The figure shows three views and two pictorial views of one solid part (mm, origin at its lowest corner). Answer the questions. Coordinates: 2 decimals unless noted, no trailing zeros. Loops run counter-clockwise (first coordinate to the right, second up) from the corner with the lowest first, then second, coordinate; pieces in that order, holes last.
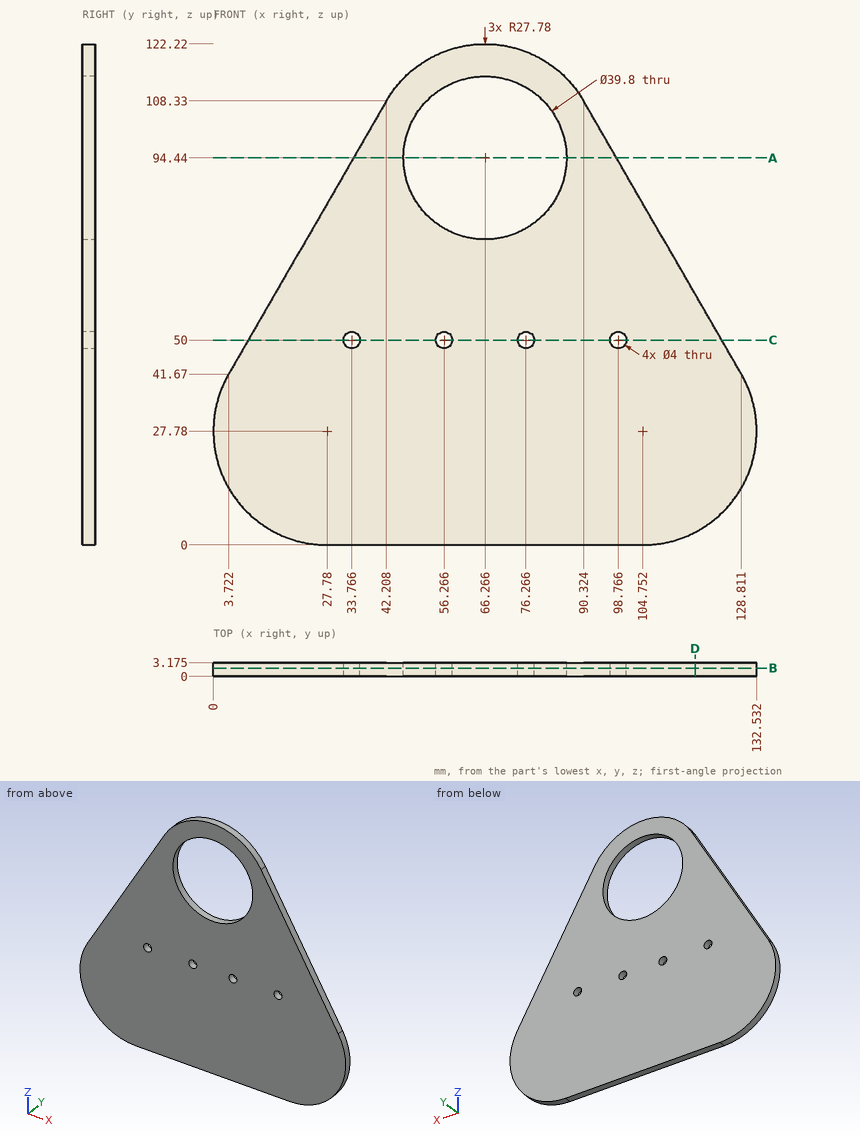
Q1. A cutting plane is placed at A-A (z = 94.44). Give the vertices of the cut face in (x, y) (1 decimal).
Findings below:
outline: (34.2, 0) - (46.4, 0) - (46.4, 3.2) - (34.2, 3.2) - close; (86.2, 0) - (98.3, 0) - (98.3, 3.2) - (86.2, 3.2) - close
Q2. A flat-ended cylindrical pin translates along its axis: pin 1 Ø1.5 at (x, y) = (74.5, 1.5) entering from +Z. Find the tip coordinate at first contact, or state that the pin passes through.
Findings below:
pin 1: stops at z = 121.19
Q3. A cutting plane is placed at C-C (z = 50). Give the vertices of the cut face in (x, y) (1 decimal), then the cut area to 3 significant figures.
Findings below:
outline: (8.5, 0) - (31.8, 0) - (31.8, 3.2) - (8.5, 3.2) - close; (35.8, 0) - (54.3, 0) - (54.3, 3.2) - (35.8, 3.2) - close; (58.3, 0) - (74.3, 0) - (74.3, 3.2) - (58.3, 3.2) - close; (78.3, 0) - (96.8, 0) - (96.8, 3.2) - (78.3, 3.2) - close; (100.8, 0) - (124, 0) - (124, 3.2) - (100.8, 3.2) - close
area: 316 mm2
Q4. Straight lines are drawn through the part: probe 1 along X at (y, z) = (2.4, 50) (1 decimal); probe 2 along Z at (x, y) = (67, 2.65); probe 3 along X at (y, z) = (0.1, 112) (1 decimal). For each, find the intervals that lie inside material, in ascending order.
Findings below:
probe 1: x = 8.5 to 31.8, 35.8 to 54.3, 58.3 to 74.3, 78.3 to 96.8, 100.8 to 124
probe 2: z = 0 to 74.55, 114.33 to 122.21
probe 3: x = 44.7 to 56.9, 75.6 to 87.8
Q5. A cutting plane is placed at B-B (y = 1.9). Give the vertices of the cut face in (x, z) (1 decimal), then the cut area to 3 significant figures.
Findings below:
outline: (3.7, 41.7) arc R27.8 ccw to (27.8, 0) - (104.8, 0) arc R27.8 ccw to (128.8, 41.7) - (90.3, 108.3) arc R27.8 ccw to (42.2, 108.3) - close; hole circle Ø4 at (33.8, 50); hole circle Ø39.8 at (66.3, 94.4); hole circle Ø4 at (56.3, 50); hole circle Ø4 at (76.3, 50); hole circle Ø4 at (98.8, 50)
area: 10,100 mm2
Q6. A cutting plane is placed at D-D (x = 117.5). Give the vertices of the cut face in (y, z) (1 decimal), then the cut area to 3 significant figures.
Findings below:
outline: (0, 3.1) - (3.2, 3.1) - (3.2, 61.3) - (0, 61.3) - close
area: 185 mm2
